Here's how the part is built. I have some questions about the finished solid (model axes, mm). Face numbers are marked on the shaded views. A direction names the side the tool comes from. Coordinates: 2 decimals unless noted, no trailing zeros. Write each loop counter-clockwise with the first axis right and the second up, starting at its lowest first coordinate (ties: lowest second). Pieces come first, ordered by that corner, then holes.
Item 1: I want a section at D-D (z = 40.5). Please give me the cut outline in (x, y) (3 decimals), and give its area (3 significant figures).
Item 2: I want a section at C-C (x = -39). Please give me the cut outline in (y, z) (3 decimals).
Item 3: I want a section at A-A (y = 12.7). Please give me the cut outline in (x, z) (3 decimals).
Item 4: For the marked faces 1 and 2, which set-ups out of +Z, -Z, +X, -X, +Y, -Y let a thin tool reach every point of the face, with its end or its side?
Item 5: I want a section at B-B (x = -64). Please give me the cut outline in (y, z) (3 decimals), and give its area (3 significant figures).
Item 6: Please list where these lines run through material, in increasing order: line 1 (Z direction, x = -16.5, y = 15.5) (3 decimals); line 2 (Y direction, x = -66.5, z = 68.5) (3 decimals); line 3 (Z direction, x = -35.5, y = 1.5).
Item 7: I'm going to push flat-ended pins straight in: P1, Ø10.5, axis at x = -43.899, y = 12.7, coming from the +Z side (3 decimals); P2, Ø5, axis at x = -70.5, z = 30.5, coming from the +Y side (3 decimals). Where does each tip first touch, or does it pass through?
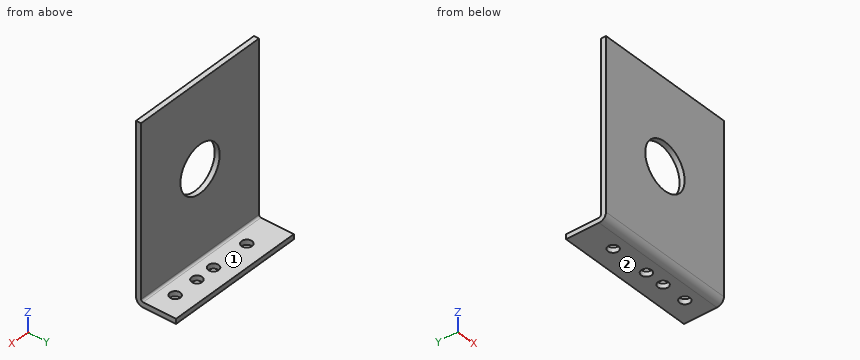
Autodesk Inventor part; units mm, degrees
ref_plane "YZ Plane" through (0, 0, 0) normal (1, 0, 0) x (0, 1, 0)
ref_plane "XZ Plane" through (0, 0, 0) normal (0, 1, 0) x (-1, 0, 0)
ref_plane "XY Plane" through (0, 0, 0) normal (0, 0, 1) x (1, 0, 0)
sketch "Sketch3" plane through (0, 0, 0) normal (0, 1, 0) x (-1, 0, 0)
  line L0 (0, 0) -> (90, 0)
  line L1 (90, 0) -> (90, 86.54)
  line L2 (90, 86.54) -> (0, 86.54)
  line L3 (0, 86.54) -> (0, 0)
  line L4 (0, 0) -> (0, -25.4)
  line L5 (0, -25.4) -> (90, -25.4)
  line L6 (90, -25.4) -> (90, 0)
  dimension "d13" = 90
  dimension "d14" = 86.54
  dimension "d15" = 25.4
extrude "Plate3" add sketch "Sketch3" along normal blind 3.175
sketch "Sketch4" plane through (-90, 0, -22.225) normal (0, 0, -1) x (-1, 0, 0)
  line L0 (-90, 0) -> (0, 0)
  line L1 (0, 0) -> (0, 25.4)
  line L2 (0, 25.4) -> (-90, 25.4)
  line L3 (-90, 25.4) -> (-90, 0)
edge flange "Flange2" height 25.4 angle 90 thickness 3.175 bend radius 1.27 thickness toward (0, 0, -1) relief tear relief width 3.175 relief depth 1.5875 edges at (-45, 3.175, -25.4) wall of the first edge with corners at (0, 0, -22.225) (-90, 0, -22.225) (-90, 25.4, -22.225) (0, 25.4, -22.225)
bend "Bend2"
corner "Corner2"
sketch "Sketch5" plane through (0, 3.175, 0) normal (0, 1, 0) x (1, 0, 0)
  line L0 (0, 20.955) -> (-90, 20.955)
  line L1 (-90, -86.54) -> (-90, 20.955)
  line L2 (0, -86.54) -> (-90, -86.54)
  line L3 (0, 20.955) -> (0, -86.54)
  line L4 (-45, 20.955) -> (-45, -86.54)
  line L5 (0, -32.7925) -> (-90, -32.7925)
  circle A0 centre (-45, -32.7925) radius 15
  point P0 (0, 0)
  dimension "d27" = 30
extrude "Cut1" cut sketch "Sketch5" against normal blind 3.175 contours A0 L5 L4 | L4 L5 A0 | A0 L4 L5 | L4 A0 L5
sketch "Sketch6" plane through (-90, 25.4, -22.225) normal (0, 0, 1) x (1, 0, 0)
  circle A0 centre (20.701, -12.7) radius 3.302
  circle A1 centre (58.801, -12.7) radius 3.302
  circle A2 centre (46.101, -12.7) radius 3.302
  circle A3 centre (1.651, -12.7) radius 3.302
  circle A4 centre (119.9021, -12.7) radius 3.302
  circle A5 centre (75.4521, -12.7) radius 3.302
  point P0 (90, -25.4)
extrude "Cut2" cut sketch "Sketch6" against normal blind 3.175 contours A0 | A1 | A2 | A5
equation "\"d28\" = Thickness"
equation "\"d30\" = Thickness"
equation "\"d17\" = BendReliefWidth"
equation "\"d18\" = BendReliefDepth"
equation "\"d19\" = MinimumRemnant"
equation "\"d20\" = BendRadius"
equation "\"d24\" = CornerReliefSize"
equation "\"d25\" = GapSize"
equation "\"d26\" = JacobiRadiusSize"
equation "\"BendRadius\" = Thickness"
equation "\"BendReliefWidth\" = Thickness"
equation "\"BendReliefDepth\" = 0.5 * Thickness"
equation "\"CornerReliefSize\" = 4 * Thickness"
equation "\"MinimumRemnant\" = 2 * Thickness"
equation "\"TransitionRadius\" = BendRadius"
equation "\"JacobiRadiusSize\" = BendRadius"
equation "\"GapSize\" = Thickness"
equation "\"d2\" = BendRadius"
equation "\"d16\" = BendRadius"
properties part number "New Bracket for arm motor"
Answer:
1. outline: (-90, 0) - (-57.868, 0) - (-57.868, 3.175) - (-90, 3.175) - close; (-32.132, 0) - (0, 0) - (0, 3.175) - (-32.132, 3.175) - close
1. area: 204 mm2
2. outline: (0, -20.955) arc R4.445 ccw to (4.445, -25.4) - (25.4, -25.4) - (25.4, -22.225) - (4.445, -22.225) arc R1.27 cw to (3.175, -20.955) - (3.175, 19.045) - (0, 19.045) - close; (0, 46.54) - (3.175, 46.54) - (3.175, 86.54) - (0, 86.54) - close
3. outline: (-90, -25.4) - (-72.601, -25.4) - (-72.601, -22.225) - (-90, -22.225) - close; (-65.997, -25.4) - (-47.201, -25.4) - (-47.201, -22.225) - (-65.997, -22.225) - close; (-40.597, -25.4) - (-34.501, -25.4) - (-34.501, -22.225) - (-40.597, -22.225) - close; (-27.897, -25.4) - (-17.85, -25.4) - (-17.85, -22.225) - (-27.897, -22.225) - close; (-11.246, -25.4) - (0, -25.4) - (0, -22.225) - (-11.246, -22.225) - close
4. face 1: +Z, +X, -X, +Y
4. face 2: -Z, +X, -X, +Y, -Y
5. outline: (0, -20.955) arc R4.445 ccw to (4.445, -25.4) - (25.4, -25.4) - (25.4, -22.225) - (4.445, -22.225) arc R1.27 cw to (3.175, -20.955) - (3.175, 86.54) - (0, 86.54) - close
5. area: 422 mm2
6. line 1: z = -25.4 to -22.225
6. line 2: y = 0 to 3.175
6. line 3: z = -24.28 to 21.18, 44.4 to 86.54
7. P1: stops at z = -22.225
7. P2: stops at y = 3.175
